```python
from build123d import *

# Parameters (mm, degrees)
F1_DEPTH  = 40
F1_FACE_W = 30
F1_FACE_H = 20
F3_DEPTH  = 22


with BuildPart() as f1:
    # F0 (on Front) → F1 (new body)
    with BuildSketch(Plane.XZ):
        Polygon((0, 20), (0, 0), (30, 0), (30, 8), (18, 20), align=None)
        Polygon((18, 20), (30, 8), (30, 20), align=None)
    extrude(amount=-F1_DEPTH)

    # F2 (on Front) + F1_face (on face) → F3 (cut)
    with BuildSketch(Plane.XZ):
        Polygon((30, 20), (18, 20), (30, 8), align=None)
    with BuildSketch(Plane(origin=(15, 40, 10), x_dir=(1, 0, 0), z_dir=(0, 1, 0))):
        Rectangle(F1_FACE_W, F1_FACE_H)
    extrude(amount=-F3_DEPTH, dir=(0, -1, 0), mode=Mode.SUBTRACT)


solid = f1.part
```
Verification items for the finished model (mm, model axes). A direction names the side the tool comes from. Round coordinates to 2 decimals unless told otherwise and drop trailing zeros. Write each loop counter-clockwise with the first axis right and the second up, starting at its lowest first coordinate (ties: lowest second). Pieces come first, ordered by that corner, then holes.
1. Section check C-C on y = 6.5. Enter the section's corners in (x, z), plus the area to 3 significant figures.
2. Gauge pin test, flat end, axial feed: P1, Ø1.5, axis at x = 9, y = 21.5, coming from the -Z side. Record the tip position at first contact, or that the pin passes through.
3. Section check B-B on x = 22. Enter the section's corners in (y, z).
4. Scan lines: L1, parallel to Z at x = 21, y = 18.5; L2, parallel to Z at x = 20.25, y = 4.5; L3, parallel to X at y = 3, z = 11.75. Record each from-to range of solid material in increasing order.
5. Section check A-A on z = 14.5. Enter the section's corners in (x, y).
6. Access from +Z, -Z, +X, -X, +Y, -Y to the whole of each face (thin tool, end or side, straight path). Record for faces 1 (the flat face through (0, 20, 10)), 2 (the flat face through (24, 11, 14)).
Answer:
1. outline: (0, 0) - (30, 0) - (30, 8) - (18, 20) - (0, 20) - close
1. area: 528 mm2
2. P1: stops at z = 0
3. outline: (0, 0) - (40, 0) - (40, 20) - (22, 20) - (22, 16) - (0, 16) - close
4. L1: z = 0 to 17
4. L2: z = 0 to 17.75
4. L3: x = 0 to 26.25
5. outline: (0, 0) - (23.5, 0) - (23.5, 22) - (30, 22) - (30, 40) - (0, 40) - close
6. face 1: +Z, -Z, -X, +Y, -Y
6. face 2: +Z, +X, -Y
